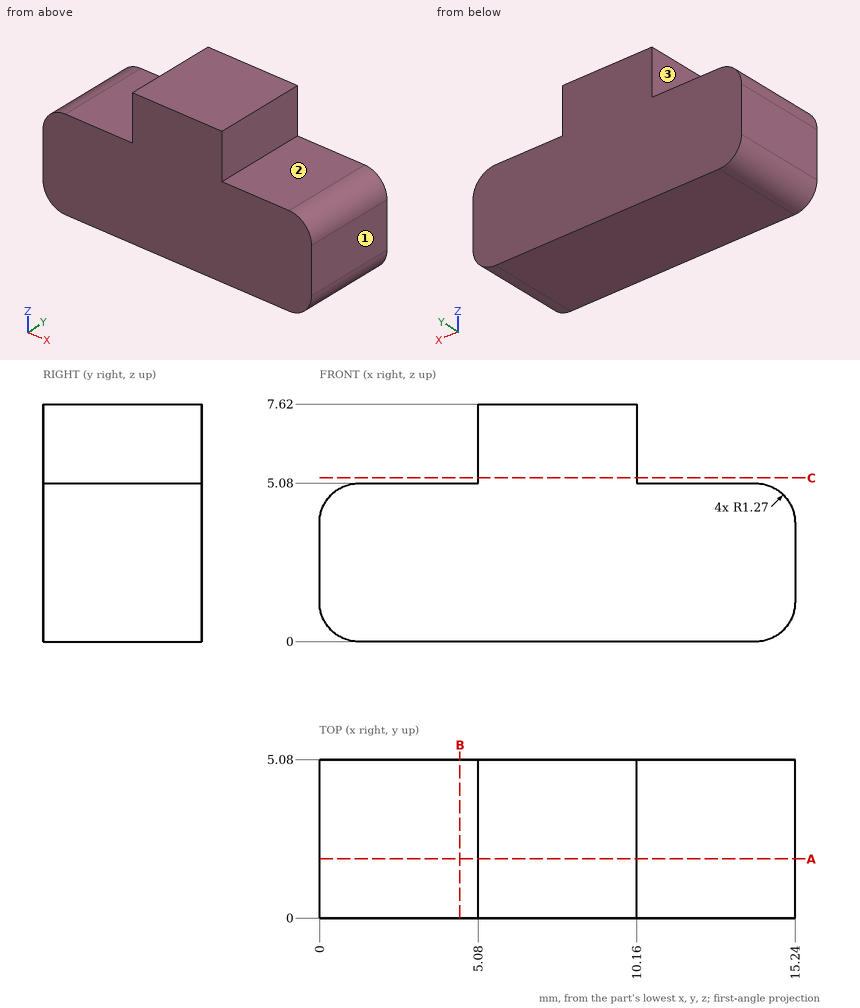
Answer from the drawing. Dimensions are ordinates in mm from the lowest x, y and z of the part. A direction names the side the tool comes from. Coordinates: 2 decimals unless noted, no trailing zeros. Loops run counter-clockwise (first coordinate to the right, second up) from the corner with the lowest first, then second, coordinate; pieces in that order, holes last.
1) For the marked faces 1, 2 and 3, determine the directions among +Z, -Z, +X, -X, +Y, -Y from which every point of the face is accessible in a straight line to the end or side of a thin tool.
Results:
face 1: +Z, -Z, +X, +Y, -Y
face 2: +Z, +X, +Y, -Y
face 3: +Z, -X, +Y, -Y
2) Consider probe 1 along Z at (x, y) = (12.5, 3.45); probe 2 along X at (y, z) = (4.05, 6.5); probe 3 along X at (y, z) = (4.4, 4.5). Determine where each line is inside the solid, lowest interval first.
Results:
probe 1: z = 0 to 5.08
probe 2: x = 5.08 to 10.16
probe 3: x = 0.2 to 15.04
3) Flat-ended cylindrical pins translate along their axes: pin 1 (1.5 mm diameter, centred on x = 1.5, y = 4.5, fed in from -Z); pin 2 (1.1 mm diameter, centred on x = 4, y = 2, fed in from +Z); pin 3 (0.8 mm diameter, centred on y = 3, z = 6.5, fed in from -X); pin 4 (1.3 mm diameter, centred on y = 3, z = 6, fed in from +X). Find the tip coordinate at first contact, or state that the pin passes through.
Results:
pin 1: stops at z = 0
pin 2: stops at z = 5.08
pin 3: stops at x = 5.08
pin 4: stops at x = 10.16
4) Section B-B (x = 4.5) is taken. Give the vertices of the cut face in (y, z), plus the area to 3 significant figures.
Results:
outline: (0, 0) - (5.08, 0) - (5.08, 5.08) - (0, 5.08) - close
area: 25.8 mm2
5) Section C-C (z = 5.25) is taken. Give the vertices of the cut face in (x, y), plus the area to 3 significant figures.
Results:
outline: (5.08, 0) - (10.16, 0) - (10.16, 5.08) - (5.08, 5.08) - close
area: 25.8 mm2
6) Section A-A (y = 1.9) is taken. Give the vertices of the cut face in (x, z), plus the area to 3 significant figures.
Results:
outline: (0, 1.27) arc R1.27 ccw to (1.27, 0) - (13.97, 0) arc R1.27 ccw to (15.24, 1.27) - (15.24, 3.81) arc R1.27 ccw to (13.97, 5.08) - (10.16, 5.08) - (10.16, 7.62) - (5.08, 7.62) - (5.08, 5.08) - (1.27, 5.08) arc R1.27 ccw to (0, 3.81) - close
area: 88.9 mm2
